Source: CAD feature listing. Evaluate the final solid. Frame: model axes, mm. A direction names the side the tool comes from. Give positions to 0.01 mm unless a question says otherwise; leave off trailing zeros. Write each loop counter-clockwise with the first axis right and the second up, starting at its lowest first coordinate (ties: lowest second). Pieces come first, ordered by that corner, then holes.
```python
from build123d import *

# Parameters (mm, degrees)
F0_W     = 127
F0_H     = 76.2
F1_DEPTH = 38.1
F2_R     = 6.35
F3_DEPTH = 50.8
F4_R     = 5.08
F5_W     = 114.3
F5_H     = 50.8
F6_DEPTH = 31.75
F7_SIZE  = 5.08


with BuildPart() as f1:
    # F0 (on Front) → F1 (new body)
    with BuildSketch(Plane.XZ):
        Rectangle(F0_W, F0_H)
    extrude(amount=F1_DEPTH)

    # F2 (on Front) → F3 (cut)
    with BuildSketch(Plane.XZ):
        Circle(F2_R)
    extrude(amount=F3_DEPTH, mode=Mode.SUBTRACT)

    # F4
    f4_edges = [f1.edges().sort_by_distance(p)[0] for p in [
        (63.5, 0, 0),
        (0, 0, -38.1),
        (-63.5, 0, 0),
    ]]
    fillet(f4_edges, radius=F4_R)

    # F5 (on Front) → F6 (cut)
    with BuildSketch(Plane.XZ):
        Rectangle(F5_W, F5_H)
    extrude(amount=F6_DEPTH, mode=Mode.SUBTRACT)

    # F7
    f7_edges = [f1.edges().sort_by_distance(p)[0] for p in [
        (-6.35, -31.75, 0),
        (0, -31.75, 25.4),
        (57.15, -31.75, 0),
        (-57.15, -31.75, 0),
        (0, -31.75, -25.4),
    ]]
    chamfer(f7_edges, length=F7_SIZE)


solid = f1.part
```
1. Cut plane D-D, the plane y = -3.5. Return the cut outline in (x, z), then the cut area to 3 significant figures.
2. Mould query, pull axis Z, two halves, no side actions, for faces 1 (the flat face through (57.15, -13, 0)), 2 (the cylindrical face through (0.889, -1.528, -36.651)), 3 (the flat face through (-1, -19, 38.1)), 4 (the flat face through (-12, -31.75, 0)). Classes: +Z half, -Z half, draft (parallel to the pull), parting line (faces both ways), or undercut.
3. Access query for faces 5 (the flat face through (54.57, -29.25, -0.36)), 6 (the cylindrical face through (-1.38, -37.46, -6.2)). Directions: +Z, -Z, +X, -X, +Y, -Y. A direction counts if a zero-diameter tool reaches every point of the face in a straight line with its end or side. Return the directions, or none.
4. Line query: L1, parallel to X at y = -37, z = 0; L2, parallel to Z at x = -48.5, y = -26; L3, parallel to Z at x = 0, y = -37.2. Output: solid intervals per line, ascending.
5. Cut plane B-B, the plane y = -29. Return the cut outline in (x, z), then the cut area to 3 significant figures.
6. Cut plane C-C, the plane x = 41.5. Return the cut outline in (y, z), then the cut area to 3 significant figures.
7. Cut plane A-A, the plane x = 0. Return the cut outline in (y, z), then the cut area to 3 significant figures.
8. Contact query for a flat-ended pin moving along its axis: P1, Ø8, axis at x = -31, z = 16.5, coming from the +Y side. Output: stop coordinate, or through.
Response values:
1. outline: (-63.25, -37.85) - (63.25, -37.85) - (63.25, 38.1) - (-63.25, 38.1) - close; hole (-57.15, -25.4) - (57.15, -25.4) - (57.15, 25.4) - (-57.15, 25.4) - close
1. area: 3,800 mm2
2. face 1: undercut
2. face 2: -Z half
2. face 3: +Z half
2. face 4: undercut
3. face 5: +Y
3. face 6: +Y, -Y
4. L1: x = -63.5 to -6.35, 6.35 to 63.5
4. L2: z = -38.1 to -25.4, 25.4 to 38.1
4. L3: z = -38.1 to -6.35, 6.35 to 38.1
5. outline: (-63.5, -38.1) - (63.5, -38.1) - (63.5, 38.1) - (-63.5, 38.1) - close; hole (-54.82, -23.07) - (54.82, -23.07) - (54.82, 23.07) - (-54.82, 23.07) - close
5. area: 4,620 mm2
6. outline: (-38.1, -38.1) - (-5.08, -38.1) arc R5.08 ccw to (0, -33.02) - (0, -25.4) - (-26.67, -25.4) - (-31.75, -20.32) - (-31.75, 20.32) - (-26.67, 25.4) - (0, 25.4) - (0, 38.1) - (-38.1, 38.1) - close
6. area: 1,310 mm2
7. outline: (-38.1, -38.1) - (-5.08, -38.1) arc R5.08 ccw to (0, -33.02) - (0, -25.4) - (-26.67, -25.4) - (-31.75, -20.32) - (-31.75, -11.43) - (-36.83, -6.35) - (-38.1, -6.35) - close; (-38.1, 6.35) - (-36.83, 6.35) - (-31.75, 11.43) - (-31.75, 20.32) - (-26.67, 25.4) - (0, 25.4) - (0, 38.1) - (-38.1, 38.1) - close
7. area: 1,200 mm2
8. P1: stops at y = -31.57
